Could you check a few things on this model? Use its own coordinates, in mm. A direction names the side the tool comes from. Round coordinates to 2 decimals unless told otherwise and drop trailing zeros. Loops run counter-clockwise (first coordinate to the right, second up) from the corner with the lowest first, then second, coordinate; pieces in that order, holes last. Notation, with made-up numbers: (6.25, 76) -> (22.25, 76) arc R26 ccw to (22.25, 115) -> close; hole circle Ø3 at (54, 36.5). An arc over 180 degrees is marked (long way). Put each result on its own line as item: value. Start each with the question number.
1. Imagine slicing it at D-D, the plane z = 10. Count the separate pieces of the cut face and the enclosed holes in it, and give its area (3 significant figures).
2. Imagine slicing it at B-B, the plane x = -12.5. Please give me the cut outline in (y, z).
3. If we mould it in two halves opening along Z, with no side actions, what happens to faces 1 (the flat face through (-50, 49, 28.4)), 2 (the cylindrical face through (-49.5, -46.07, 15)), 3 (the cylindrical face through (45.633, 52.859, 11.341))? For each: pulls with the +Z half, pulls with the -Z half, needs draft (parallel to the pull), parting line crosses it, or undercut.
4. I need wall thicknesses on line 1 (Y direction, x = 25.25, z = 9.25); line 2 (Y direction, x = 50.25, z = 12); line 3 (Y direction, x = -25, z = 10). Which ranges of each line are inside material? Lowest first, please. Write a range as [from, to].
5. I'm going to push flat-ended pins straight in: P1, Ø1, axis at x = 56.5, z = 27, coming from the -Y side; P2, Ø0.7, axis at y = 53.5, z = 27, coming from the +X side; P3, Ø5.5, axis at x = 42.4, z = 10, coming from the +Y side. Where does each tip first touch, or does it pass through?
6. Which directions (+Z, -Z, +X, -X, +Y, -Y) give clear straight access to the entire face, cutting with the end or side of a thin tool? Please do faces 4 (the flat face through (58, -1, 20)), 5 (the flat face through (59, 37.75, 28)), 6 (the cylindrical face through (50.17, 43.75, 15.03)), 7 (the flat face through (46.73, 50, 10)), 8 (the flat face through (-61, 12.75, 26)).
```python
from build123d import *

# Parameters (mm, degrees)
CYLINDER007_R              = 3.5
CYLINDER007_DEPTH          = 8
CYLINDER007_ROLL_ANGLE     = -90
CYLINDER008_R              = 0.6
CYLINDER008_DEPTH          = 11
PRISM001_DEPTH             = 10
PRISM001_ROLL_ANGLE        = 90.00003
PRISM001_PITCH_ANGLE       = -30.000033
PRISM001_PLACEMENT_ANGLE   = -8e-06
BOX015_W                   = 10
BOX015_H                   = 18
BOX015_DEPTH               = 20
BOX016_W                   = 10
BOX016_H                   = 11
BOX016_DEPTH               = 15
BOX017_W                   = 10
BOX017_H                   = 25
BOX017_DEPTH               = 12
BOX018_W                   = 8.5
BOX018_H                   = 4
BOX018_DEPTH               = 7
BOX019_W                   = 8
BOX019_H                   = 4
BOX019_DEPTH               = 10.5
BOX020_W                   = 8.5
BOX020_H                   = 4
BOX020_DEPTH               = 7
BOX021_W                   = 13
BOX021_H                   = 4
BOX021_DEPTH               = 8
BOX022_W                   = 10
BOX022_H                   = 8.5
BOX022_DEPTH               = 8
BOX023_W                   = 5
BOX023_H                   = 14
BOX023_DEPTH               = 9
BOX024_W                   = 43
BOX024_H                   = 4
BOX024_DEPTH               = 19
SKETCH104_R                = 1.4
EXTRUDE093_DEPTH           = 12
BOX014_W                   = 10
BOX014_H                   = 56.75
BOX014_DEPTH               = 12
EXTRUDE092_DEPTH           = 30
EXTRUDE091_DEPTH           = 30
SKETCH101_R                = 4
SKETCH101_R_2              = 1.4
SKETCH101_R_3              = 2.25
EXTRUDE090_DEPTH           = 27.4
BOX026_W                   = 13
BOX026_H                   = 3
BOX026_DEPTH               = 15
EXTRUDE094_DEPTH           = 2.5
SKETCH100_W                = 47
SKETCH100_H                = 15
EXTRUDE089_DEPTH           = 2
EXTRUDE089_ROLL_ANGLE      = -0.000172
EXTRUDE089_PITCH_ANGLE     = -0.040176
EXTRUDE089_PLACEMENT_ANGLE = 2.8e-05


with BuildPart() as cylinder007:
    # Cylinder007 → Cylinder007 (new body)
    with BuildSketch(Plane.XY):
        Circle(CYLINDER007_R)
    extrude(amount=CYLINDER007_DEPTH)


with BuildPart() as cylinder007_1:
    # Cylinder007 roll: moved
    add(cylinder007.part.rotate(Axis((0, 0, 0), (1, 0, 0)), CYLINDER007_ROLL_ANGLE))


with BuildPart() as cylinder007_2:
    # Cylinder007 placement: moved
    add(cylinder007_1.part.moved(Location((42.4, 48, 10))))


with BuildPart() as cylinder008:
    # Cylinder008 → Cylinder008 (new body)
    with BuildSketch(Plane(origin=(46.125, 51.85, 17), x_dir=(1, 0, 0), z_dir=(0, 0, 1))):
        Circle(CYLINDER008_R)
    extrude(amount=CYLINDER008_DEPTH)


with BuildPart() as fusion035005:
    # Prism001 → Prism001 (new body)
    with BuildSketch(Plane.XY):
        Polygon((5, 0), (2.5, 4.330127), (-2.5, 4.330127), (-5, 0), (-2.5, -4.330127), (2.5, -4.330127), align=None)
    extrude(amount=PRISM001_DEPTH)


with BuildPart() as fusion035005_1:
    # Prism001 roll: moved
    add(fusion035005.part.rotate(Axis((0, 0, 0), (1, 0, 0)), PRISM001_ROLL_ANGLE))


with BuildPart() as fusion035005_2:
    # Prism001 pitch: moved
    add(fusion035005_1.part.rotate(Axis((0, 0, 0), (0, 1, 0)), PRISM001_PITCH_ANGLE))


with BuildPart() as fusion035005_3:
    # Prism001 placement: moved
    add(fusion035005_2.part.moved(Location((42.4, 51.75, 10))).rotate(Axis((42.4, 51.75, 10), (0, 0, 1)), PRISM001_PLACEMENT_ANGLE))

    # Fusion035005: union Cylinder007, Cylinder008
    add(cylinder007_2.part)
    add(cylinder008.part)


with BuildPart() as cube015:
    # Box015 → Box015 (new body)
    with BuildSketch(Plane(origin=(-67, 15.5, 8.5), x_dir=(1, 0, 0), z_dir=(0, 0, 1))):
        with Locations((5, 9)):
            Rectangle(BOX015_W, BOX015_H)
    extrude(amount=BOX015_DEPTH)


with BuildPart() as cube016:
    # Box016 → Box016 (new body)
    with BuildSketch(Plane(origin=(54, -25, 12), x_dir=(1, 0, 0), z_dir=(0, 0, 1))):
        with Locations((5, 5.5)):
            Rectangle(BOX016_W, BOX016_H)
    extrude(amount=BOX016_DEPTH)


with BuildPart() as cube017:
    # Box017 → Box017 (new body)
    with BuildSketch(Plane(origin=(54, -14, 15), x_dir=(1, 0, 0), z_dir=(0, 0, 1))):
        with Locations((5, 12.5)):
            Rectangle(BOX017_W, BOX017_H)
    extrude(amount=BOX017_DEPTH)


with BuildPart() as cube018:
    # Box018 → Box018 (new body)
    with BuildSketch(Plane(origin=(32.75, 51, 20), x_dir=(1, 0, 0), z_dir=(0, 0, 1))):
        with Locations((4.25, 2)):
            Rectangle(BOX018_W, BOX018_H)
    extrude(amount=BOX018_DEPTH)


with BuildPart() as cube019:
    # Box019 → Box019 (new body)
    with BuildSketch(Plane(origin=(19, 51, 16.5), x_dir=(1, 0, 0), z_dir=(0, 0, 1))):
        with Locations((4, 2)):
            Rectangle(BOX019_W, BOX019_H)
    extrude(amount=BOX019_DEPTH)


with BuildPart() as cube020:
    # Box020 → Box020 (new body)
    with BuildSketch(Plane(origin=(-45.9, 51, 20), x_dir=(1, 0, 0), z_dir=(0, 0, 1))):
        with Locations((4.25, 2)):
            Rectangle(BOX020_W, BOX020_H)
    extrude(amount=BOX020_DEPTH)


with BuildPart() as cube021:
    # Box021 → Box021 (new body)
    with BuildSketch(Plane(origin=(0.75, 51, 19.5), x_dir=(1, 0, 0), z_dir=(0, 0, 1))):
        with Locations((6.5, 2)):
            Rectangle(BOX021_W, BOX021_H)
    extrude(amount=BOX021_DEPTH)


with BuildPart() as cube022:
    # Box022 → Box022 (new body)
    with BuildSketch(Plane(origin=(54, 26.5, 20), x_dir=(1, 0, 0), z_dir=(0, 0, 1))):
        with Locations((5, 4.25)):
            Rectangle(BOX022_W, BOX022_H)
    extrude(amount=BOX022_DEPTH)


with BuildPart() as cube023:
    # Box023 → Box023 (new body)
    with BuildSketch(Plane(origin=(57, 23.75, 18.25), x_dir=(1, 0, 0), z_dir=(0, 0, 1))):
        with Locations((2.5, 7)):
            Rectangle(BOX023_W, BOX023_H)
    extrude(amount=BOX023_DEPTH)


with BuildPart() as cube024:
    # Box024 → Box024 (new body)
    with BuildSketch(Plane(origin=(-35, -56, 8), x_dir=(1, 0, 0), z_dir=(0, 0, 1))):
        with Locations((21.5, 2)):
            Rectangle(BOX024_W, BOX024_H)
    extrude(amount=BOX024_DEPTH)


with BuildPart() as extrude093:
    # Sketch104 → Extrude093 (new body)
    with BuildSketch(Plane.XY.offset(27)):
        with Locations((-60, 46.5)):
            Circle(SKETCH104_R)
        with Locations((57.75, 46.5)):
            Circle(SKETCH104_R)
        with Locations((-60, -46.5)):
            Circle(SKETCH104_R)
        with Locations((57.75, -46.5)):
            Circle(SKETCH104_R)
    extrude(amount=-EXTRUDE093_DEPTH)


with BuildPart() as fusion035003:
    # Box014 → Box014 (new body)
    with BuildSketch(Plane(origin=(-67, -44, 15), x_dir=(1, 0, 0), z_dir=(0, 0, 1))):
        with Locations((5, 28.375)):
            Rectangle(BOX014_W, BOX014_H)
    extrude(amount=BOX014_DEPTH)

    # Fusion035003: union Cube015, Cube016, Cube017, Cube018, Cube019, Cube020, Cube021, Cube022, Cube023, Cube024, Extrude093
    add(cube015.part)
    add(cube016.part)
    add(cube017.part)
    add(cube018.part)
    add(cube019.part)
    add(cube020.part)
    add(cube021.part)
    add(cube022.part)
    add(cube023.part)
    add(cube024.part)
    add(extrude093.part)


with BuildPart() as fusion035003_1:
    # Fusion035003 placement: moved
    add(fusion035003.part.moved(Location((0, 0, 5))))


with BuildPart() as extrude092:
    # Sketch103 → Extrude092 (new body)
    with BuildSketch(Plane.XY):
        Polygon((53.5, -52.25), (-56.5, -52.25), (-57.5, -51.25), (-57.5, 50.75), (-56.5, 51.75), (53.5, 51.75), (55, 50.25), (55, -50.75), align=None)
    extrude(amount=EXTRUDE092_DEPTH)


with BuildPart() as cut008:
    # Sketch102 → Extrude091 (new body)
    with BuildSketch(Plane.XY):
        Polygon((54.25, -54.5), (-57.25, -54.5), (-65.25, -46.5), (-65.25, 46), (-57.25, 54), (54.25, 54), (61.25, 47), (61.25, -47.5), align=None)
    extrude(amount=EXTRUDE091_DEPTH)

    # Cut007: cut Extrude092
    add(extrude092.part, mode=Mode.SUBTRACT)


with BuildPart() as cut008_1:
    # Cut007 placement: moved
    add(cut008.part.moved(Location((0, 0, 2))))

    # Cut008: cut Fusion035003
    add(fusion035003_1.part, mode=Mode.SUBTRACT)


with BuildPart() as extrude090:
    # Sketch101 → Extrude090 (new body)
    with BuildSketch(Plane.XY):
        with Locations((25.25, -42.25)):
            Circle(SKETCH101_R)
        with Locations((25.25, -42.25)):
            Circle(SKETCH101_R_2, mode=Mode.SUBTRACT)
        with Locations((53.25, -51.25)):
            Circle(SKETCH101_R_3)
        with BuildLine():
            Line((-53.75, 52.75), (-46.75, 52.75))
            Line((-46.75, 52.75), (-46.75, 47.25))
            ThreePointArc((-53.75, 47.25), (-50.25, 43.75), (-46.75, 47.25))
            Line((-53.75, 47.25), (-53.75, 52.75))
        make_face()
        with Locations((-50.25, 47.25)):
            Circle(SKETCH101_R_2, mode=Mode.SUBTRACT)
        with BuildLine():
            Line((46.75, 52.75), (53.75, 52.75))
            Line((53.75, 52.75), (53.75, 47.25))
            ThreePointArc((46.75, 47.25), (50.25, 43.75), (53.75, 47.25))
            Line((46.75, 47.25), (46.75, 52.75))
        make_face()
        with Locations((50.25, 47.25)):
            Circle(SKETCH101_R_2, mode=Mode.SUBTRACT)
        with BuildLine():
            Line((-53.75, -52.75), (-46.75, -52.75))
            Line((-46.75, -52.75), (-46.75, -47.25))
            ThreePointArc((-46.75, -47.25), (-50.25, -43.75), (-53.75, -47.25))
            Line((-53.75, -47.25), (-53.75, -52.75))
        make_face()
        with Locations((-50.25, -47.25)):
            Circle(SKETCH101_R_2, mode=Mode.SUBTRACT)
    extrude(amount=EXTRUDE090_DEPTH)


with BuildPart() as extrude090_1:
    # Extrude090 placement: moved
    add(extrude090.part.moved(Location((0, 0, 1))))


with BuildPart() as cube026:
    # Box026 → Box026 (new body)
    with BuildSketch(Plane(origin=(34, 48.75, 2), x_dir=(1, 0, 0), z_dir=(0, 0, 1))):
        with Locations((6.5, 1.5)):
            Rectangle(BOX026_W, BOX026_H)
    extrude(amount=BOX026_DEPTH)


with BuildPart() as extrude094:
    # Sketch105 → Extrude094 (new body)
    with BuildSketch(Plane.YZ):
        Polygon((0, 0), (0, 5), (-5, 5), (-2.5, 0), align=None)
    extrude(amount=EXTRUDE094_DEPTH)


with BuildPart() as extrude094_1:
    # Extrude094 placement: moved
    add(extrude094.part.moved(Location((43, 52, 16))))


with BuildPart() as obj1:
    # Sketch100 → Extrude089 (new body)
    with BuildSketch(Plane.XY):
        Polygon((54.25, -54.5), (-57.25, -54.5), (-65.25, -46.5), (-65.25, 46), (-57.25, 54), (54.25, 54), (61.25, 47), (61.25, -47.5), align=None)
        with Locations((-13.25, -43)):
            Rectangle(SKETCH100_W, SKETCH100_H, mode=Mode.SUBTRACT)
    extrude(amount=EXTRUDE089_DEPTH)


with BuildPart() as obj1_1:
    # Extrude089 roll: moved
    add(obj1.part.rotate(Axis((0, 0, 0), (1, 0, 0)), EXTRUDE089_ROLL_ANGLE))


with BuildPart() as obj1_2:
    # Extrude089 pitch: moved
    add(obj1_1.part.rotate(Axis((0, 0, 0), (0, 1, 0)), EXTRUDE089_PITCH_ANGLE))


with BuildPart() as obj1_3:
    # Extrude089 placement: moved
    add(obj1_2.part.rotate(Axis((0, 0, 0), (0, 0, 1)), EXTRUDE089_PLACEMENT_ANGLE))

    # Fusion035002: union Extrude090, Cube026, Extrude094
    add(extrude090_1.part)
    add(cube026.part)
    add(extrude094_1.part)

    # Fusion035004: union Cut008
    add(cut008_1.part)

    # Cut009: cut Fusion035005
    add(fusion035005_3.part, mode=Mode.SUBTRACT)


solid = obj1_3.part
```
Entries:
1. separate pieces: 2
1. enclosed holes: 4
1. area: 2,100 mm^2
2. outline: (-54.5, -0.01) -> (-50.5, -0.01) -> (-50.5, 1.99) -> (-54.5, 1.99) -> close; (-54.5, 2) -> (-52.25, 2) -> (-52.25, 13) -> (-54.5, 13) -> close; (-35.5, -0.01) -> (54, -0.01) -> (54, 1.99) -> (-35.5, 1.99) -> close; (51.75, 2) -> (54, 2) -> (54, 32) -> (51.75, 32) -> close
3. face 1: pulls with the +Z half
3. face 2: needs draft
3. face 3: undercut
4. line 1: [-54.5, -52.25], [-46.25, -43.65], [-40.85, -38.25], [51.75, 54]
4. line 2: [-54.5, -52.25], [43.75, 45.85], [48.65, 54]
4. line 3: [-54.5, -52.25], [51.75, 54]
5. P1: y = -52.75
5. P2: x = 55.1
5. P3: y = -52.25
6. face 4: +Z, +X, -X
6. face 5: +Z, +X
6. face 6: +Z
6. face 7: none
6. face 8: +Z, -X
